```python
from build123d import *

# Parameters (mm, degrees)
CYLINDER2790_R     = 38
CYLINDER2790_DEPTH = 30
BOX969_W           = 2
BOX969_H           = 6
BOX969_DEPTH       = 6
BOX970_W           = 2
BOX970_H           = 6
BOX970_DEPTH       = 6
BOX971_W           = 2
BOX971_H           = 6
BOX971_DEPTH       = 6
BOX972_W           = 2
BOX972_H           = 6
BOX972_DEPTH       = 6
BOX973_W           = 2
BOX973_H           = 6
BOX973_DEPTH       = 6
BOX968_W           = 2
BOX968_H           = 6
BOX968_DEPTH       = 6
TUBE123_R          = 21
TUBE123_R_2        = 2
TUBE123_DEPTH      = 64
TUBE124_R          = 25
TUBE124_R_2        = 2
TUBE124_DEPTH      = 26
BOX891_W           = 30
BOX891_H           = 64
BOX891_DEPTH       = 18


with BuildPart() as obj1:
    # Cylinder2790 → Cylinder2790 (new body)
    with BuildSketch(Plane.XY):
        Circle(CYLINDER2790_R)
    extrude(amount=CYLINDER2790_DEPTH)


with BuildPart() as krychle968:
    # Box969 → Box969 (new body)
    with BuildSketch(Plane(origin=(-12, -4, 10), x_dir=(1, 0, 0), z_dir=(0, 0, 1))):
        with Locations((1, 3)):
            Rectangle(BOX969_W, BOX969_H)
    extrude(amount=BOX969_DEPTH)


with BuildPart() as krychle969:
    # Box970 → Box970 (new body)
    with BuildSketch(Plane(origin=(10, 26, 10), x_dir=(1, 0, 0), z_dir=(0, 0, 1))):
        with Locations((1, 3)):
            Rectangle(BOX970_W, BOX970_H)
    extrude(amount=BOX970_DEPTH)


with BuildPart() as krychle970:
    # Box971 → Box971 (new body)
    with BuildSketch(Plane(origin=(-12, 26, 10), x_dir=(1, 0, 0), z_dir=(0, 0, 1))):
        with Locations((1, 3)):
            Rectangle(BOX971_W, BOX971_H)
    extrude(amount=BOX971_DEPTH)


with BuildPart() as krychle971:
    # Box972 → Box972 (new body)
    with BuildSketch(Plane(origin=(10, 12, 10), x_dir=(1, 0, 0), z_dir=(0, 0, 1))):
        with Locations((1, 3)):
            Rectangle(BOX972_W, BOX972_H)
    extrude(amount=BOX972_DEPTH)


with BuildPart() as krychle972:
    # Box973 → Box973 (new body)
    with BuildSketch(Plane(origin=(-12, 12, 10), x_dir=(1, 0, 0), z_dir=(0, 0, 1))):
        with Locations((1, 3)):
            Rectangle(BOX973_W, BOX973_H)
    extrude(amount=BOX973_DEPTH)


with BuildPart() as compound1242:
    # Box968 → Box968 (new body)
    with BuildSketch(Plane(origin=(10, -4, 10), x_dir=(1, 0, 0), z_dir=(0, 0, 1))):
        with Locations((1, 3)):
            Rectangle(BOX968_W, BOX968_H)
    extrude(amount=BOX968_DEPTH)

    # Compound1242: union Krychle968, Krychle969, Krychle970, Krychle971, Krychle972
    add(krychle968.part)
    add(krychle969.part)
    add(krychle970.part)
    add(krychle971.part)
    add(krychle972.part)


with BuildPart() as tube123:
    # Tube123 → Tube123 (new body)
    with BuildSketch(Plane(origin=(0, 61, 37), x_dir=(1, 0, 0), z_dir=(0, -1, 0))):
        Circle(TUBE123_R)
        Circle(TUBE123_R_2, mode=Mode.SUBTRACT)
    extrude(amount=TUBE123_DEPTH)


with BuildPart() as tube124:
    # Tube124 → Tube124 (new body)
    with BuildSketch(Plane(origin=(0, -3, 37), x_dir=(1, 0, 0), z_dir=(0, -1, 0))):
        Circle(TUBE124_R)
        Circle(TUBE124_R_2, mode=Mode.SUBTRACT)
    extrude(amount=TUBE124_DEPTH)


with BuildPart() as common:
    # Box891 → Box891 (new body)
    with BuildSketch(Plane(origin=(-15, -17, 11), x_dir=(1, 0, 0), z_dir=(0, 0, 1))):
        with Locations((15, 32)):
            Rectangle(BOX891_W, BOX891_H)
    extrude(amount=BOX891_DEPTH)

    # Cut977: cut Tube124
    add(tube124.part, mode=Mode.SUBTRACT)

    # Cut001: cut Tube123
    add(tube123.part, mode=Mode.SUBTRACT)

    # Cut1048: cut Compound1242
    add(compound1242.part, mode=Mode.SUBTRACT)

    # Common: intersect obj1
    add(obj1.part, mode=Mode.INTERSECT)


solid = common.part
```
Design review of the part built by this model. Coordinates are the model's own, in mm. A direction names the side the tool comes from. Coordinates: 2 decimals unless noted, no trailing zeros. Write each loop counter-clockwise with the first axis right and the second up, starting at its lowest first coordinate (ties: lowest second). Pieces come first, ordered by that corner, then holes.
1) To check wall thickness, follow L1, parallel to Z at x = -0.5, y = -1; L2, parallel to X at y = 24, z = 21; L3, parallel to X at y = 19, z = 18.75. State the ranges of each line that lie inside material, in increasing order.
2) Add section C-C (x = 11). Write out the cut boundary in (y, z).
3) Add section B-B (z = 20.5). Write out the cut boundary in (x, y).
4) Add section A-A (y = 15). Write out the cut boundary in (x, z), plus the area to 3 significant figures.
5) Machinability: for faces 1 (the flat face through (-11, -4, 13)), 2 (the flat face through (0, -3, 15)), 3 (the flat face through (-11, 26, 13)), which of the approach directions +Z, -Z, +X, -X, +Y, -Y give a long, thin tool a straight path to every point of the face, cutting with its end or side? Answer none if there is none.
6) Add section D-D (z = 13.5). State how many separate pieces and enclosed holes the cut face has, plus the area to 3 significant figures.
7) Mouldability with a two-part tool opening along X and no side actions: class faces 4 (the cylindrical face through (0, 38, 14)), 5 (the flat face through (-15, 9, 17)), 6 (the flat face through (-10, 15, 13)) as +X half, -X half, draft (parallel to the pull), parting line (faces both ways), or undercut.
8) Insertion check: pin 1 (3 mm diameter, centred on x = -8.5, z = 19.5, fed in from -Y); pin 2 (4 mm diameter, centred on x = 5.5, z = 15, fed in from -Y); pin 3 (1.6 mm diameter, centred on x = -11, y = 29, fed in from -Z); pin 4 (0.6 mm diameter, centred on x = 10.5, z = 12.5, fed in from +Y). Each pin has a flat end and moves straight along its axis. Give the tip position at first contact, or say it passes through.
Check result:
1. L1: z = 11 to 16.01
1. L2: x = -15 to -13.6, 13.6 to 15
1. L3: x = -15 to -10.39, 10.39 to 15
2. outline: (-17, 11) - (-4, 11) - (-4, 14.55) - (-17, 14.55) - close; (-3, 16) - (2, 16) - (2, 11) - (12, 11) - (12, 16) - (18, 16) - (18, 11) - (26, 11) - (26, 16) - (32, 16) - (32, 11) - (36.37, 11) - (36.37, 19.11) - (-3, 19.11) - close
3. outline: (-15, -3) - (-12.99, -3) - (-12.99, 35.71) arc R38 ccw to (-15, 34.91) - close; (12.99, -3) - (15, -3) - (15, 34.91) arc R38 ccw to (12.99, 35.71) - close
4. outline: (-15, 11) - (-12, 11) - (-12, 16) - (-10, 16) - (-10, 11) - (10, 11) - (10, 16) - (12, 16) - (12, 11) - (15, 11) - (15, 22.3) arc R21 cw to (-15, 22.3) - close
4. area: 189 mm2
5. face 1: +Z, -Z
5. face 2: +Z, -Y
5. face 3: -Z
6. separate pieces: 1
6. enclosed holes: 6
6. area: 1,310 mm2
7. face 4: parting line
7. face 5: -X half
7. face 6: undercut
8. pin 1: passes through
8. pin 2: stops at y = -3
8. pin 3: stops at z = 16
8. pin 4: stops at y = 36.61
